Design review of the part built by this model. Coordinates are the model's own, in mm. A direction names the side the tool comes from. Round coordinates to 2 decimals unless told otherwise and drop trailing zeros. Write each loop counter-clockwise with the first axis right and the second up, starting at its lowest first coordinate (ties: lowest second). Pieces come first, ordered by that corner, then holes. Notation, with made-up numbers: (77.25, -38) - (113.25, -38) arc R28 ccw to (113.25, -10) - close; hole circle Ø6 at (66.5, 38.5). An arc over 180 degrees is marked (long way). Use one line per item in the form item = value.
Autodesk Inventor part; units mm, degrees
ref_plane "Plano de trabajo3" through (0, 0, -52) normal (0, 0, 1) x (1, 0, 0)
ref_plane "YZ Plane" through (0, 0, 0) normal (1, 0, 0) x (0, 1, 0)
ref_plane "XZ Plane" through (0, 0, 0) normal (0, 1, 0) x (-1, 0, 0)
sketch "Boceto1" plane through (0, 0, 0) normal (0, 0, 1) x (1, 0, 0)
  arc A0 (11.6645, -103.4622) -> (0, -112.3475) centre (12.4952, -116.6519) ccw construction
  line L0 (-152.4797, 0) -> (132.3175, 0) construction
  line L1 (0, 89.2085) -> (0, -112.3475) construction
  circle A1 centre (0, 0) radius 17.5
  dimension "d0" = 35
extrude "Extrusión1" add sketch "Boceto1" along normal blind 30
ref_plane "Plano de trabajo1" through (0, 0, -30) normal (0, 0, 1) x (1, 0, 0)
sketch "Boceto2" plane through (0, 0, -30) normal (0, 0, 1) x (1, 0, 0)
  circle A0 centre (0, 0) radius 42.5
  dimension "d4" = 85
loft "Solevación1" add profiles "Boceto2" section 2 edges at (-17.5, 0, 0)
ref_plane "Plano de trabajo2" through (0, 0, -55) normal (0, 0, 1) x (1, 0, 0)
sketch "Boceto3" plane through (0, 0, -55) normal (0, 0, 1) x (1, 0, 0)
  circle A0 centre (0, 0) radius 42.5
  dimension "d10" = 85
loft "Solevación2" add profiles "Boceto3" section 2 edges at (-42.5, 0, -30)
shell "Vaciado1" thickness 3 outward yes removed faces 2 at (-10.6049, 7.3037, -55) at (4.865, -5.1831, 30)
ref_plane "Plano de trabajo3" through (0, 0, -52) normal (0, 0, 1) x (1, 0, 0)
sketch "Boceto4" plane through (0, 0, -52) normal (0, 0, 1) x (1, 0, 0)
  circle A0 centre (0, 0) radius 48.5
  dimension "d17" = 97
extrude "Extrusión2" add sketch "Boceto4" against normal blind 14
sketch "Boceto5" plane through (0, 0, -66) normal (0, 0, -1) x (-1, 0, 0)
  circle A0 centre (0, 0) radius 45.5
  dimension "d20" = 91
extrude "Extrusión3" cut sketch "Boceto5" against normal blind 12
sketch "Boceto6" plane through (0, 0, -54) normal (0, 0, -1) x (-1, 0, 0)
  circle A0 centre (0, 0) radius 42.5
  dimension "d23" = 85
extrude "Extrusión4" cut sketch "Boceto6" against normal blind 12
sketch "Boceto7" plane through (0, 0, 30) normal (0, 0, 1) x (1, 0, 0)
  point P0 (0, 0)
properties part number "CAPSULA 2DA MITAD"
Q1. To check wall thickness, follow line 1 along Y through (x, z) = (0, -39); line 2 along Y through (x, z) = (0, 19.5); line 3 along X through (y, z) = (-15.5, -8). State the ranges of each line that lie inside material, in increasing order. Write a range as from..to.
Calculated:
line_1 = -45.5..-42.5, 42.5..45.5
line_2 = -20.5..-17.5, 17.5..20.5
line_3 = -23.4..-18.54, 18.54..23.4
Q2. We need section C-C on z = -34. Write out the cut boundary in (x, y).
Calculated:
outline = circle Ø91 at (0, 0); hole circle Ø85 at (0, 0)
Q3. Draft analysis for pull direction X (two halves, no side actions). For faces 4 (the conical face through (10.181, 19.574, -0.791)), 5 (the flat face through (15.1, 9.2, 30)), 6 (the flat face through (14, 41, -54)), state which applies: released by +X, released by -X, zero draft, split by the parting line, or undercut.
Calculated:
face_4 = split by the parting line
face_5 = zero draft
face_6 = undercut
Q4. We need section B-B on z = 9.5. Write out the cut boundary in (x, y).
Calculated:
outline = circle Ø41 at (0, 0); hole circle Ø35 at (0, 0)
Q5. Machinability: for faces 1 (the cylindrical face through (-4.444, 20.013, 15.341)), 2 (the cylindrical face through (36.107, -27.686, -60.084)), 3 (the flat face through (-14.6, 43.3, -66)), which of the approach directions +Z, -Z, +X, -X, +Y, -Y give a long, thin tool a straight path to every point of the face, cutting with its end or side? Answer none if there is none.
Calculated:
face_1 = +Z
face_2 = -Z
face_3 = -Z, +X, -X, +Y, -Y
Q6. For P1, Ø12, axis at x = -31.5, y = -9.5, coming from the -Z side; P2, Ø12, axis at x = -24.5, y = -34.5, coming from the +Z side; P3, Ø4, axis at y = 1.5, z = -13.5, coming from the -X side, all flat-tipped, find the tip position at first contact; note any pin that passes through.
Calculated:
P1 = -25.68
P2 = -17.89
P3 = -34.29
Q7. We need section A-A on x = 0. Write out the cut boundary in (y, z).
Calculated:
outline = (-48.5, -66) - (-45.5, -66) - (-45.5, -54) - (-42.5, -54) - (-42.5, -30) - (-17.5, 0) - (-17.5, 30) - (-20.5, 30) - (-20.5, 1.09) - (-45.5, -28.91) - (-45.5, -52) - (-48.5, -52) - close; (17.5, 0) - (42.5, -30) - (42.5, -54) - (45.5, -54) - (45.5, -66) - (48.5, -66) - (48.5, -52) - (45.5, -52) - (45.5, -28.91) - (20.5, 1.09) - (20.5, 30) - (17.5, 30) - close
